Input: part model. Units: mm. Frame: model coordinates. Give positions to 0.01 mm unless a question says otherwise; leave off trailing zeros. Loops run counter-clockwise (first coordinate to the right, second up) from the corner with the lowest first, then second, coordinate; pieces in that order, holes last. Notation, with made-up numbers: M -36.5,86.5 L -15.5,86.5 A13 ccw -15.5,109.5 Z; hole C 88,-21.75 d2. An arc over 180 degrees is marked long. One line per item, written item: value. Start each with the question number.
(1) Section B-B on y = 11.75. Output: boundary loops of the cut face in (x, z), plus the area to 3 significant figures.
(2) Section A-A on z = 1.3. Output: boundary loops of the cut face in (x, y).
(3) Ray query, line 1 along Y through (x, z) = (42.5, 1.45); line 2 along Y through (x, z) = (3.5, 0.5); line 3 along Y through (x, z) = (3, 0.6). Return the intervals inside material, ascending. Write a range as from..to.
```python
from build123d import *

# Parameters (mm, degrees)
F0_W     = 50
F0_H     = 25
F1_DEPTH = 3
F3_D     = 3.2
F5_DEPTH = 25


with BuildPart() as f1:
    # F0 (on Top) → F1 (new body)
    with BuildSketch(Plane.XY):
        with Locations((25, 11.048387)):
            Rectangle(F0_W, F0_H)
    extrude(amount=F1_DEPTH)

    # F3 (through all)
    with Locations(Plane.XY.offset(3)):
        with Locations((2.12132, 21.427067), (47.87868, 21.427067), (47.87868, 0.669707), (2.12132, 0.669707)):
            Hole(F3_D / 2)

    # F4 (on face) → F5 (cut)
    with BuildSketch(Plane.XY.offset(3)):
        Polygon((50, 7.048387), (50, 11.048387), (50, 15.048387), (42, 15.048387), (42, 7.048387), align=None)
    extrude(amount=-F5_DEPTH, mode=Mode.SUBTRACT)


solid = f1.part
```
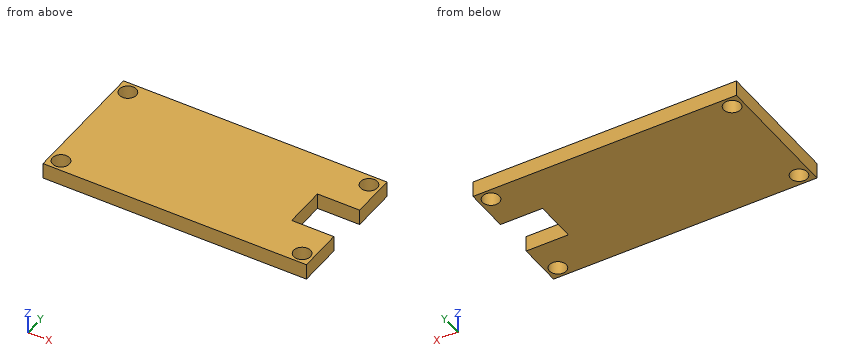
Output values:
1. outline: M 0,0 L 42,0 L 42,3 L 0,3 Z
1. area: 126 mm²
2. outline: M 0,-1.45 L 50,-1.45 L 50,7.05 L 42,7.05 L 42,15.05 L 50,15.05 L 50,23.55 L 0,23.55 Z; hole C 2.12,0.67 d3.2; hole C 2.12,21.43 d3.2; hole C 47.88,0.67 d3.2; hole C 47.88,21.43 d3.2
3. line 1: y = -1.45..7.05, 15.05..23.55
3. line 2: y = -1.45..-0.14, 1.48..20.62, 22.24..23.55
3. line 3: y = -1.45..-0.67, 2.01..20.09, 22.76..23.55
